```python
from build123d import *
from build123d.topology import SkipClean

# Parameters (mm, degrees)
SKETCH2_W               = 67.5
SKETCH2_H               = 32.75
BOSS_EXTRUDE1_DEPTH     = 21.25
CUT_EXTRUDE3_DEPTH      = 52.606080068
CUT_EXTRUDE3_DEPTH_BACK = 0.05
SKETCH4_W               = 7.5
SKETCH4_H               = 32.7
CUT_EXTRUDE6_DEPTH      = 0.05
SKETCH5_W               = 7.5
SKETCH5_H               = 65.45
CUT_EXTRUDE7_DEPTH      = 0.05
SKETCH6_W               = 7.119941604
SKETCH6_H               = 65.013736252
BOSS_EXTRUDE9_DEPTH     = 0.05
SKETCH15_W              = 6.895148233
SKETCH15_H              = 32.7
BOSS_EXTRUDE14_DEPTH    = 0.01
SKETCH16_W              = 7.139794156
SKETCH16_H              = 65.046080354
BOSS_EXTRUDE15_DEPTH    = 0.01
SKETCH18_W              = 12
SKETCH18_H              = 15
CUT_EXTRUDE14_DEPTH     = 3
CUT_EXTRUDE14_DRAFT     = -30
SKETCH19_W              = 7.508639757
SKETCH19_H              = 3.271964709
BOSS_EXTRUDE16_DEPTH    = 3
SKETCH21_R              = 2.5
CUT_EXTRUDE17_DEPTH     = 2
CUT_EXTRUDE17_DRAFT     = -35


with BuildPart() as part:
    # Sketch2 → Boss-Extrude1 (new body)
    with BuildSketch(Plane(origin=(0, 0, 0), x_dir=(0, 0, -1), z_dir=(1, 0, 0))):
        Rectangle(SKETCH2_W, SKETCH2_H)
    extrude(amount=BOSS_EXTRUDE1_DEPTH)

    # Sketch3 → Cut-Extrude3 (cut, two sides: drawn at the far end of the back side and taken through both)
    with SkipClean():  # the faces are left unmerged after this step: merging them gives an invalid solid
        with BuildSketch(Plane(origin=(0, 16.375, 0), x_dir=(1, 0, 0), z_dir=(0, 1, 0)).offset(-CUT_EXTRUDE3_DEPTH_BACK)):
            with BuildLine():
                Line((-134.022457335, 33.75), (13.75, 33.75))
                Line((13.75, 33.75), (13.751, 33.75))
                Line((13.75, 33.75), (13.75, -31.747079321))
                Line((13.75, -31.747079321), (21.25, -31.747079321))
                Line((21.25, -31.747079321), (169.022457335, -31.747079321))
                Line((169.022457335, -31.747079321), (231.45697941, 257.127853894))
                Line((231.45697941, 257.127853894), (-71.58793526, 322.624933215))
                Line((-71.58793526, 322.624933215), (-134.022457335, 33.75))
            make_face()
        extrude(amount=CUT_EXTRUDE3_DEPTH + CUT_EXTRUDE3_DEPTH_BACK, mode=Mode.SUBTRACT)
    add(part.part.scale(1), mode=Mode.REPLACE)  # the faces are merged on a copy

    # Sketch4 → Cut-Extrude6 (cut)
    with BuildSketch(Plane(origin=(0, 0, -33.75), x_dir=(-1, 0, 0), z_dir=(0, 0, -1))):
        with Locations((-17.5, -0.025)):
            Rectangle(SKETCH4_W, SKETCH4_H)
    extrude(amount=-CUT_EXTRUDE6_DEPTH, mode=Mode.SUBTRACT)

    # Sketch5 → Cut-Extrude7 (cut)
    with BuildSketch(Plane(origin=(0, -16.375, 0), x_dir=(-1, 0, 0), z_dir=(0, -1, 0))):
        with Locations((-17.5, 0.975)):
            Rectangle(SKETCH5_W, SKETCH5_H)
    extrude(amount=-CUT_EXTRUDE7_DEPTH, mode=Mode.SUBTRACT)

    # Sketch6 → Boss-Extrude9 (add)
    with BuildSketch(Plane(origin=(0, 16.325, 0), x_dir=(1, 0, 0), z_dir=(0, 1, 0))):
        with Locations((17.690029198, 1.193131874)):
            Rectangle(SKETCH6_W, SKETCH6_H)
    extrude(amount=BOSS_EXTRUDE9_DEPTH)

    # Sketch15 → Boss-Extrude14 (add)
    with BuildSketch(Plane(origin=(0, 0, -33.7), x_dir=(-1, 0, 0), z_dir=(0, 0, -1))):
        with Locations((-17.802425883, 0.025)):
            Rectangle(SKETCH15_W, SKETCH15_H)
    extrude(amount=BOSS_EXTRUDE14_DEPTH)

    # Sketch16 → Boss-Extrude15 (add)
    with BuildSketch(Plane(origin=(0, -16.325, 0), x_dir=(-1, 0, 0), z_dir=(0, -1, 0))):
        with Locations((-17.680102922, 1.186959823)):
            Rectangle(SKETCH16_W, SKETCH16_H)
    extrude(amount=BOSS_EXTRUDE15_DEPTH)


with BuildPart() as cut_extrude14_tool:
    # Sketch18 → Cut-Extrude14 (with draft: the straight prism first)
    with BuildSketch(Plane.ZY):
        with Locations((-26.267087013, 5.422853248)):
            Rectangle(SKETCH18_W, SKETCH18_H)
    extrude(amount=-CUT_EXTRUDE14_DEPTH)
    # Cut-Extrude14: the draft: its side faces are tilted about the plane it starts from
    cut_extrude14_sides = [cut_extrude14_tool.faces().sort_by_distance(p)[0] for p in [
        (1.5, 5.422853248, -32.267087013),
        (1.5, -2.077146752, -26.267087013),
        (1.5, 5.422853248, -20.267087013),
        (1.5, 12.922853248, -26.267087013),
    ]]
    draft(cut_extrude14_sides, Plane.ZY, CUT_EXTRUDE14_DRAFT)


with BuildPart() as part_1:
    add(part.part)

    # Cut-Extrude14: cut by cut_extrude14_tool
    add(cut_extrude14_tool.part, mode=Mode.SUBTRACT)

    # Sketch19 → Boss-Extrude16 (add)
    with BuildSketch(Plane.ZY.offset(-3)):
        with Locations((-26.237986877, 8.548870353)):
            Rectangle(SKETCH19_W, SKETCH19_H)
    extrude(amount=BOSS_EXTRUDE16_DEPTH)


with BuildPart() as cut_extrude17_tool:
    # Sketch21 → Cut-Extrude17 (with draft: the straight prism first)
    with BuildSketch(Plane(origin=(0, 0, -33.75), x_dir=(-1, 0, 0), z_dir=(0, 0, -1))):
        with Locations((-10.25, -10.875)):
            Circle(SKETCH21_R)
    extrude(amount=-CUT_EXTRUDE17_DEPTH)
    # Cut-Extrude17: the draft: its side faces are tilted about the plane it starts from
    cut_extrude17_sides = [cut_extrude17_tool.faces().sort_by_distance(p)[0] for p in [
        (12.75, -10.875, -32.75),
    ]]
    draft(cut_extrude17_sides, Plane(origin=(0, 0, -33.75), x_dir=(-1, 0, 0), z_dir=(0, 0, -1)), CUT_EXTRUDE17_DRAFT)


with BuildPart() as part_2:
    add(part_1.part)

    # Cut-Extrude17: cut by cut_extrude17_tool
    add(cut_extrude17_tool.part, mode=Mode.SUBTRACT)


solid = part_2.part
```
Model file for the job. Use its own axes, mm. A direction names the side the tool comes from. Coordinates: 2 decimals unless noted, no trailing zeros. Write each loop counter-clockwise with the first axis right and the second up, starting at its lowest first coordinate (ties: lowest second). Pieces come first, ordered by that corner, then holes. Notation, with made-up numbers: (79, -35) - (135, -35) arc R13 ccw to (135, -26) - close; hole circle Ø6 at (22.25, -37). An arc over 180 degrees is marked (long way). One line per item, written item: value. Start each with the question number.
1. Tool access for faces 1 (the flat face through (18, 16.375, -1)), 2 (the flat face through (10, -11, -31.75)), 3 (the flat face through (2, 10.185, -26)): list every direction of +Z, -Z, +X, -X, +Y, -Y with a clear straight run to the whole face (end or side of a thin tool).
2. Probe line 1 (Y direction, x = 20.25, z = -10) (3 decimals); line 2 (Z direction, x = 14.75, y = 15); line 3 (X direction, y = 1.5, z = -28). List the from-to ranges inside material, lowest first. Write a range as from..to.
3. Flat gauge pins, fed straight in: pin 1 (1.1 mm diameter, centred on x = 10, y = -11.5, fed in from -Z); pin 2 (8 mm diameter, centred on x = 18.5, z = -8, fed in from -Y) (3 decimals); pin 3 (8 mm diameter, centred on x = 18, y = -5, fed in from -Z). Where does each tip first touch, or does it go through?
4. Mould opens along Z. For faces 4 (the flat face through (2, 6.913, -26)), 5 (the flat face through (6, 16.375, 0)), 6 (the flat face through (7, 0, -33.75)) say: released by +Z, released by -Z, zero draft, split by the parting line, or undercut.
5. Slice it at A-A (z = -26). Write the cut outline in (x, y) (3 decimals), plus the area to 3 significant figures.
Answers below:
1. face 1: +Z, -Z, +X, -X, +Y
1. face 2: -Z
1. face 3: -X
2. line 1: y = -16.335..16.375
2. line 2: z = -33.71..33.75
2. line 3: x = 3..21.25
3. pin 1: stops at z = -31.93
3. pin 2: stops at y = -16.335
3. pin 3: stops at z = -33.71
4. face 4: undercut
4. face 5: zero draft
4. face 6: released by -Z
5. outline: (0, -16.375) - (13.75, -16.375) - (13.75, -16.325) - (14.11, -16.325) - (14.11, -16.335) - (21.25, -16.335) - (21.25, 16.375) - (14.13, 16.375) - (14.13, 16.325) - (13.75, 16.325) - (13.75, 16.375) - (0, 16.375) - (0, 12.923) - (3, 11.191) - (3, 10.185) - (0, 10.185) - (0, 6.913) - (3, 6.913) - (3, -0.345) - (0, -2.077) - close
5. area: 666 mm^2
